```python
from build123d import *

# Parameters (mm, degrees)
SKETCH1_W                    = 44.45
SKETCH1_H                    = 1980.184
BOSS_EXTRUDE1_DEPTH          = 44.45
SKETCH2_W                    = 38.1
SKETCH2_H                    = 38.1
CUT_EXTRUDE1_DEPTH           = 1981.807518913
CUT_EXTRUDE2_DEPTH           = 993.085567612
SKETCH13_R                   = 3.3734375
CUT_EXTRUDE7_DEPTH           = 992.338449567
F_10_0_1935_DIAMETER_HOLE1_D = 4.9149


with BuildPart() as part:
    # Sketch1 → Boss-Extrude1 (new body)
    with BuildSketch(Plane.XY):
        Rectangle(SKETCH1_W, SKETCH1_H)
    extrude(amount=BOSS_EXTRUDE1_DEPTH)

    # Sketch2 → Cut-Extrude1 (cut, through all)
    with BuildSketch(Plane(origin=(0, 990.092, 0), x_dir=(1, 0, 0), z_dir=(0, 1, 0))):
        with Locations((0, -22.225)):
            Rectangle(SKETCH2_W, SKETCH2_H)
    extrude(amount=-CUT_EXTRUDE1_DEPTH, mode=Mode.SUBTRACT)

    # Sketch3 → Cut-Extrude2 (cut, through all)
    with BuildSketch(Plane(origin=(22.225, 0, 0), x_dir=(0, 0, -1), z_dir=(1, 0, 0))):
        Polygon((-44.45, 990.092), (0, 964.428780535), (0, 990.092), align=None)
        Polygon((-44.45, -990.092), (0, -964.428780535), (0, -990.092), align=None)
    extrude(amount=-CUT_EXTRUDE2_DEPTH, mode=Mode.SUBTRACT)

    # Sketch13 → Cut-Extrude7 (cut, through all)
    with BuildSketch(Plane.XY.offset(44.45)):
        with Locations((0, 939.038)):
            Circle(SKETCH13_R)
        with Locations((0, -939.038)):
            Circle(SKETCH13_R)
    extrude(amount=-CUT_EXTRUDE7_DEPTH, mode=Mode.SUBTRACT)

    # #10 (0.1935) Diameter Hole1 (through all)
    with Locations(Plane(origin=(-9.525, -612.1654, 44.45), x_dir=(1, 0, 0), z_dir=(0, 0, 1))):
        with Locations((0, 0), (19.05, 0), (0, 94.0308), (19.05, 94.0308), (0, 1130.3), (19.05, 1130.3), (0, 1224.3308), (19.05, 1224.3308)):
            Hole(F_10_0_1935_DIAMETER_HOLE1_D / 2)


solid = part.part
```
Check sheet for the modelled part. Datum: model origin and axes. Units: mm. A direction names the side the tool comes from. Round coordinates to 2 decimals unless told otherwise and drop trailing zeros. Order: outer loops, then holes, each group sorted by start corner. A loop starts at its lowest first (then second) coordinate and runs counter-clockwise, first axis right, second up.
1) Scan lines: line 1 (Z direction, x = -7, y = -286) (3 decimals); line 2 (X direction, y = 822.5, z = 34) (3 decimals); line 3 (Y direction, x = 20.5, z = 16.5). Record each from-to range of solid material in increasing order.
2) Go/stop test with a flat-tipped pin: pin 1 Ø12 at (x, z) = (10.5, 10.5) entering from -Y. Record where the tip stops, or that it passes through.
3) Tool access check on faces 1 (the flat face through (0, 14, 44.45)), 2 (the flat face through (0, 14, 41.275)). Record the directions out of +Z, -Z, +X, -X, +Y, -Y that give a thin tool (end or side, any length) a straight path to the whole face; none if there is none.
4) Section check A-A (y = -696). Record the boundary of the cut face in (x, z) (3 decimals).
5) Section check B-B (z = 10). Record the boundary of the cut face in (x, y) (3 decimals).
6) Mould release check, pull along X, two halves, no side actions. Record for faces 3 (the flat face through (22.225, -14, 22)), 4 (the flat face through (19.05, 14, 22)), 5 (the flat face through (-19.44, 977.44, 22.54)), 6 (the flat face through (-19.05, 14, 22)): +X half, -X half, draft (parallel to the pull), parting line (faces both ways), or undercut.
Result:
1. line 1: z = 0 to 3.175, 41.275 to 44.45
1. line 2: x = -22.225 to -19.05, 19.05 to 22.225
1. line 3: y = -973.96 to 973.96
2. pin 1: passes through
3. face 1: +Z, +X, -X, +Y, -Y
3. face 2: +Y, -Y
4. outline: (-22.225, 0) - (22.225, 0) - (22.225, 44.45) - (-22.225, 44.45) - close; hole (-19.05, 3.175) - (19.05, 3.175) - (19.05, 41.275) - (-19.05, 41.275) - close
5. outline: (-22.225, -970.202) - (-19.05, -970.202) - (-19.05, 970.202) - (-22.225, 970.202) - close; (19.05, -970.202) - (22.225, -970.202) - (22.225, 970.202) - (19.05, 970.202) - close
6. face 3: +X half
6. face 4: undercut
6. face 5: draft
6. face 6: undercut
